Verification items for the finished model (mm, model axes). A direction names the side the tool comes from. Round coordinates to 2 decimals unless told otherwise and drop trailing zeros. Write each loop counter-clockwise with the first axis right and the second up, starting at its lowest first coordinate (ties: lowest second). Pieces come first, ordered by that corner, then holes. Notation, with made-up numbers: (7, -26) -> (14, -26) arc R30 cw to (14, 12) -> close; hole circle Ø7 at (-10.5, 0). An arc over 180 degrees is marked (long way). Answer as a JSON object with one key per item and string values. Group by question number.
(1) Set-up check for faces 5 (the face through (-100.562, -22.418, -1.479)), 6 (the face through (-109, 54.195, 1)), 7 (the face through (-102.27, 60.95, -1.48)), 8 (the face through (-99.137, 64, -1)), 9 (the face through (-142, 8.416, 0)): record each of +Z, -Z, +X, -X, +Y, -Y from which the full face is reachable in a straight line by a thin tool's end or side.
(2) Sectioned sample at A-A on y = 19.5. Record the cut outline in (x, z), and give its area (3 significant figures).
(3) Gauge pin test, flat ends, axial feed: pin 1 Ø8.5 at (x, y) = (-108, 58.5) entering from -Z; pin 2 Ø1.8 at (y, z) = (47.5, 0) entering from -X; pin 3 Ø3.5 at (y, z) = (13, 1) entering from +X; pin 4 Ø0.9 at (y, z) = (65.5, -2) entering from +X. Record the tip position at first contact, or that the pin passes through.
(4) Scan lines: L1, parallel to Y at x = -141, z = 2.2; L2, parallel to Y at x = -124.5, z = 0.75; L3, parallel to X at y = 60.5, z = 2.4. Record each from-to range of solid material in increasing order. Write a range as from..to.
(5) Sectioned sample at D-D on z = 2. Count the separate pieces of the cut face and the enclosed holes in it, and give its area (3 significant figures).
(6) Draft check along Y on faces 1 (the face through (-116.86, -5.04, 1.48)), 2 (the face through (-136.449, 42.035, -0.042)), 3 (the face through (-109, 62, 0)), 4 (the face through (-134.1, -8.4, 0)). Enter one of: released by +Y, released by -Y, zero draft, split by the parting line, or undercut.
(7) Sectioned sample at B-B on x = -111. Record the cut outline in (y, z), and give its area (3 significant figures).
(8) Sectioned sample at C-C on y = 46.5. Record the cut outline in (x, z), and give its area (3 significant figures).
```python
from build123d import *

# Parameters (mm, degrees)
ESQUISSE1_R             = 1.7
BOSS_EXTRU_1_DEPTH      = 3
ESQUISSE2_R             = 5.2
BOSS_EXTRU_2_DEPTH      = 3
BOSS_EXTRU_2_DEPTH_BACK = 3


with BuildPart() as part:
    # Esquisse1 → Boss.-Extru.1 (new body)
    with BuildSketch(Plane.XY):
        with BuildLine():
            Line((-117.680084405, 66.939310237), (-117.680084405, 59.695120061))
            ThreePointArc((-117.680084405, 59.695120061), (-116.069171702, 55.806032765), (-112.180084405, 54.195120061))
            Line((-112.180084405, 54.195120061), (-105.294175096, 54.195120061))
            ThreePointArc((-105.294175096, 54.195120061), (-101.4050878, 52.584207358), (-99.794175096, 48.695120061))
            Line((-99.794175096, 48.695120061), (-99.794175096, 35.930823665))
            Line((-99.794175096, 35.930823665), (-99.794175096, 12.910007682))
            Line((-99.794175096, 12.910007682), (-99.794175096, 1.692208933))
            ThreePointArc((-99.794175096, 1.692208933), (-101.4050878, -2.196878364), (-105.294175096, -3.807791067))
            Line((-105.294175096, -3.807791067), (-113.390601299, -3.807791067))
            ThreePointArc((-113.390601299, -3.807791067), (-117.279688595, -5.418703771), (-118.890601299, -9.307791067))
            Line((-118.890601299, -9.307791067), (-118.890601299, -18.42196685))
            ThreePointArc((-118.890601299, -18.42196685), (-117.279688595, -22.311054147), (-113.390601299, -23.92196685))
            Line((-113.390601299, -23.92196685), (-99.794175096, -23.92196685))
            Line((-99.794175096, -23.92196685), (-99.063687308, -23.92196685))
            ThreePointArc((-99.063687308, -23.92196685), (-96.942366965, -23.043287194), (-96.063687308, -20.92196685))
            Line((-96.063687308, -20.92196685), (-96.063687308, 28.805298211))
            ThreePointArc((-96.063687308, 28.805298211), (-95.185007652, 30.926618554), (-93.063687308, 31.805298211))
            Line((-93.063687308, 31.805298211), (-89.37766128, 31.805298211))
            ThreePointArc((-89.37766128, 31.805298211), (-87.256340937, 32.683977867), (-86.37766128, 34.805298211))
            Line((-86.37766128, 34.805298211), (-86.37766128, 39.478876094))
            ThreePointArc((-86.37766128, 39.478876094), (-87.256340937, 41.600196437), (-89.37766128, 42.478876094))
            Line((-89.37766128, 42.478876094), (-93.063687308, 42.478876094))
            ThreePointArc((-93.063687308, 42.478876094), (-95.185007652, 43.35755575), (-96.063687308, 45.478876094))
            Line((-96.063687308, 45.478876094), (-96.063687308, 69.719310237))
            ThreePointArc((-96.063687308, 69.719310237), (-96.942366965, 71.840630581), (-99.063687308, 72.719310237))
            Line((-99.063687308, 72.719310237), (-112.180084405, 72.719310237))
            ThreePointArc((-112.180084405, 72.719310237), (-116.069171702, 71.108397534), (-117.680084405, 67.219310237))
            Line((-117.680084405, 67.219310237), (-117.680084405, 66.939310237))
        make_face()
        with Locations((-91.856378892, 36.719310237)):
            Circle(ESQUISSE1_R, mode=Mode.SUBTRACT)
        with Locations((-107.466378892, -14.520689763)):
            Circle(ESQUISSE1_R, mode=Mode.SUBTRACT)
        with Locations((-107.466378892, 60.719310237)):
            Circle(ESQUISSE1_R, mode=Mode.SUBTRACT)
    extrude(amount=BOSS_EXTRU_1_DEPTH)

    # Esquisse2 → Boss.-Extru.2 (add, two sides)
    with BuildSketch(Plane(origin=(0, 0, 0), x_dir=(-1, 0, 0), z_dir=(0, 0, -1))) as boss_extru_2_sk:
        with BuildLine():
            Line((121.867659056, -9.94673926), (130.584615963, -9.880075131))
            ThreePointArc((130.584615963, -9.880075131), (134.095405897, -8.402210456), (135.546378892, -4.880221341))
            Line((135.546378892, -4.880221341), (135.546378892, 5.415623015))
            ThreePointArc((135.546378892, 5.415623015), (136.425058549, 7.536943358), (138.546378892, 8.415623015))
            Line((138.546378892, 8.415623015), (145.752654566, 8.415623015))
            ThreePointArc((145.752654566, 8.415623015), (147.87397491, 9.294302671), (148.752654566, 11.415623015))
            Line((148.752654566, 11.415623015), (148.752654566, 38.179170847))
            ThreePointArc((148.752654566, 38.179170847), (147.87397491, 40.300491191), (145.752654566, 41.179170847))
            Line((145.752654566, 41.179170847), (138.546378892, 41.179170847))
            ThreePointArc((138.546378892, 41.179170847), (136.425058549, 42.057850504), (135.546378892, 44.179170847))
            Line((135.546378892, 44.179170847), (135.546378892, 52.099902349))
            ThreePointArc((135.546378892, 52.099902349), (134.081912798, 55.635436255), (130.546378892, 57.099902349))
            Line((130.546378892, 57.099902349), (120.680084405, 57.099902349))
            ThreePointArc((120.680084405, 57.099902349), (118.558764062, 57.978582005), (117.680084405, 60.099902349))
            Line((117.680084405, 60.099902349), (117.680084405, 67.719310237))
            ThreePointArc((117.680084405, 67.719310237), (116.215618311, 71.254844143), (112.680084405, 72.719310237))
            Line((112.680084405, 72.719310237), (104.136677999, 72.719310237))
            ThreePointArc((104.136677999, 72.719310237), (100.601144093, 71.254844143), (99.136677999, 67.719310237))
            Line((99.136677999, 67.719310237), (99.136677999, 59.456292263))
            ThreePointArc((99.136677999, 59.456292263), (100.601144093, 55.920758357), (104.136677999, 54.456292263))
            Line((104.136677999, 54.456292263), (126.246378892, 54.456292263))
            ThreePointArc((126.246378892, 54.456292263), (131.196126361, 52.406039732), (133.246378892, 47.456292263))
            Line((133.246378892, 47.456292263), (133.246378892, 40.977229779))
            ThreePointArc((133.246378892, 40.977229779), (134.125058549, 38.855909436), (136.246378892, 37.977229779))
            Line((136.246378892, 37.977229779), (142.162261637, 37.977229779))
            ThreePointArc((142.162261637, 37.977229779), (144.28358198, 37.098550123), (145.162261637, 34.977229779))
            Line((145.162261637, 34.977229779), (145.162261637, 14.363062522))
            ThreePointArc((145.162261637, 14.363062522), (144.28358198, 12.241742179), (142.162261637, 11.363062522))
            Line((142.162261637, 11.363062522), (136.246378892, 11.363062522))
            ThreePointArc((136.246378892, 11.363062522), (134.125058549, 10.484382866), (133.246378892, 8.363062522))
            Line((133.246378892, 8.363062522), (133.246378892, -1.293707737))
            ThreePointArc((133.246378892, -1.293707737), (131.196126361, -6.243455205), (126.246378892, -8.293707737))
            Line((126.246378892, -8.293707737), (104.136677999, -8.293707737))
            ThreePointArc((104.136677999, -8.293707737), (100.601144093, -9.758173831), (99.136677999, -13.293707737))
            Line((99.136677999, -13.293707737), (99.136677999, -18.92196685))
            ThreePointArc((99.136677999, -18.92196685), (100.601144093, -22.457500756), (104.136677999, -23.92196685))
            Line((104.136677999, -23.92196685), (113.890601299, -23.92196685))
            ThreePointArc((113.890601299, -23.92196685), (117.426135205, -22.457500756), (118.890601299, -18.92196685))
            Line((118.890601299, -18.92196685), (118.890601299, -12.946651534))
            ThreePointArc((118.890601299, -12.946651534), (119.761185096, -10.833458065), (121.867659056, -9.94673926))
        make_face()
        with Locations((107.466378892, -14.520689763)):
            Circle(ESQUISSE2_R, mode=Mode.SUBTRACT)
        with Locations((107.466378892, 60.719310237)):
            Circle(ESQUISSE2_R, mode=Mode.SUBTRACT)
    extrude(amount=BOSS_EXTRU_2_DEPTH)
    extrude(boss_extru_2_sk.sketch, amount=-BOSS_EXTRU_2_DEPTH_BACK)


solid = part.part
```
Computed values:
{
 "1": {"face 5": "-Z, +X, -Y", "face 6": "+Z, -Z", "face 7": "-Z", "face 8": "-Z, +X, +Y, -Y", "face 9": "+Z, -Z, -X, -Y"},
 "2": {"outline": "(-148.75, -3) -> (-145.16, -3) -> (-145.16, 3) -> (-148.75, 3) -> close; (-99.79, 0) -> (-96.06, 0) -> (-96.06, 3) -> (-99.79, 3) -> close", "area": "32.7 mm2"},
 "3": {"pin 1": "z = -3", "pin 2": "x = -135.55", "pin 3": "x = -96.06", "pin 4": "x = -99.14"},
 "4": {"L1": "8.42..11.36, 37.98..41.18", "L2": "-9.93..-8.29, 54.46..57.1", "L3": "-117.68..-109.15, -105.78..-96.06"},
 "5": {"separate pieces": "1", "enclosed holes": "4", "area": "1,490 mm2"},
 "6": {"face 1": "undercut", "face 2": "released by +Y", "face 3": "undercut", "face 4": "released by -Y"},
 "7": {"outline": "(-23.92, -3) -> (-18.34, -3) -> (-18.34, 0) -> (-10.71, 0) -> (-10.71, -3) -> (-8.29, -3) -> (-8.29, 0) -> (-3.81, 0) -> (-3.81, 3) -> (-23.92, 3) -> close; (54.2, 0) -> (54.46, 0) -> (54.46, -3) -> (56.9, -3) -> (56.9, 0) -> (64.53, 0) -> (64.53, -3) -> (72.72, -3) -> (72.72, 3) -> (54.2, 3) -> close", "area": "172 mm2"},
 "8": {"outline": "(-135.55, -3) -> (-133.25, -3) -> (-133.25, 3) -> (-135.55, 3) -> close; (-99.79, 0) -> (-96.06, 0) -> (-96.06, 3) -> (-99.79, 3) -> close", "area": "25.0 mm2"}
}
